Verification items for the finished model (mm, model axes). Face numbers are marked on the shaded views. Give positions to 0.01 mm unless a question says otherwise; leave off trailing zeros. Write each loop counter-clockwise with the first axis right and the second up, starting at its lowest first coordinate (ties: lowest second). Pieces come first, ordered by that corner, then holes. Notation, with made-up numbers: (-17.5, 43) - (40.5, 43) arc R20 ccw to (40.5, 47) - close; hole circle Ø2 at (-33.5, -19). An arc over 180 degrees is marked (long way). Put each result on its own line as item: value.
from build123d import *

# Parameters (mm, degrees)
F0_W     = 63.5
F0_H     = 38.1
F1_DEPTH = 6.35
F2_R     = 9.525
F3_DEPTH = 25.4


with BuildPart() as f1:
    # F0 (on Top) → F1 (new body)
    with BuildSketch(Plane.XY):
        with Locations((1.792339, 19.05)):
            Rectangle(F0_W, F0_H)
    extrude(amount=F1_DEPTH)

    # F2 (on face) → F3 (cut)
    with BuildSketch(Plane.XY.offset(6.35)):
        Polygon((-29.957661, 0), (-10.907661, 38.1), (-29.957661, 38.1), align=None)
        Polygon((33.542339, 38.1), (14.492339, 38.1), (33.542339, 0), align=None)
        with Locations((1.792339, 19.05)):
            Circle(F2_R)
    extrude(amount=-F3_DEPTH, mode=Mode.SUBTRACT)


solid = f1.part
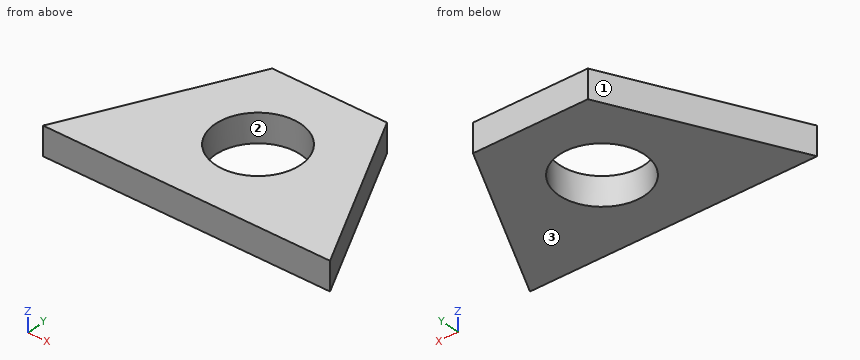
Q1. Section check B-B, the plane z = 1.75. Record the cut outline in (x, y) (3 decimals).
Answers follow:
outline: (-29.958, 0) - (33.542, 0) - (14.492, 38.1) - (-10.908, 38.1) - close; hole circle Ø19.05 at (1.792, 19.05)
Q2. Release check for a two-part mould opening along X. For the marked faces 1, 2 and 3 record: released by +X, released by -X, zero draft, split by the parting line, or undercut.
Answers follow:
face 1: released by -X
face 2: undercut
face 3: zero draft
Q3. Section check A-A, the plane y = 16.5. Record the cut outline in (x, z), plus the area to 3 significant figures.
Answers follow:
outline: (-21.71, 0) - (-7.38, 0) - (-7.38, 6.35) - (-21.71, 6.35) - close; (10.97, 0) - (25.29, 0) - (25.29, 6.35) - (10.97, 6.35) - close
area: 182 mm2
Q4. Section check D-D, the plane x = 27. Record the cut outline in (y, z), plus the area to 3 significant figures.
Answers follow:
outline: (0, 0) - (13.08, 0) - (13.08, 6.35) - (0, 6.35) - close
area: 83.1 mm2
Q5. Go/stop test with flat-tipped pins: pin 1 Ø1.5 at (x, z) = (-12.5, 5) entering from +Y; pin 2 Ø3 at (y, z) = (5.5, 1) entering from +X. Record where each tip stops, or that it passes through.
Answers follow:
pin 1: stops at y = 36.42
pin 2: stops at x = 31.54
Q6. Scan lines: line 1 along Y through (x, z) = (1.5, 5.25); line 2 along Y through (x, z) = (-6, 4.25); line 3 along X through (y, z) = (22.5, 5.25). Record each from-to range of solid material in increasing order.
Answers follow:
line 1: y = 0 to 9.53, 28.57 to 38.1
line 2: y = 0 to 13.57, 24.53 to 38.1
line 3: x = -18.71 to -7.09, 10.67 to 22.29
Q7. Section check C-C, the plane x = -4. Record the cut outline in (y, z), plus the area to 3 significant figures.
Answers follow:
outline: (0, 0) - (11.49, 0) - (11.49, 6.35) - (0, 6.35) - close; (26.61, 0) - (38.1, 0) - (38.1, 6.35) - (26.61, 6.35) - close
area: 146 mm2
